The model under review builds one solid part; all positions refer to its coordinate system, in mm. A direction names the side the tool comes from. Give positions to 0.01 mm unless a question says otherwise; leave off trailing zeros. Order: outer loops, then holes, each group sorted by start corner. A loop starts at its lowest first (then second) coordinate and runs counter-clockwise, first axis right, second up. Notation, with made-up numbers: (-28, 41) - (-13, 41) arc R10 cw to (-13, 51) - close; hole circle Ø6 at (-21, -32). An arc over 180 degrees is marked (long way). Answer as CSV lines item,"result". Start each with the question number.
from build123d import *

# Parameters (mm, degrees)
SKETCH1_W           = 50
SKETCH1_H           = 265
SKETCH1_R           = 12.5
BOSS_EXTRUDE1_DEPTH = 10
SKETCH2_W           = 50
SKETCH2_H           = 20
BOSS_EXTRUDE2_DEPTH = 30
SKETCH3_W           = 50
SKETCH3_H           = 20
BOSS_EXTRUDE3_DEPTH = 30
FILLET1_R           = 10


with BuildPart() as part:
    # Sketch1 → Boss-Extrude1 (new body)
    with BuildSketch(Plane(origin=(0, 0, 0), x_dir=(1, 0, 0), z_dir=(0, 1, 0))):
        with Locations((-25, 132.5)):
            Rectangle(SKETCH1_W, SKETCH1_H)
        with Locations(Location((-25, 240, 0), (0, 0, 270))):
            Circle(SKETCH1_R, mode=Mode.SUBTRACT)
    extrude(amount=BOSS_EXTRUDE1_DEPTH)

    # Sketch2 → Boss-Extrude2 (add)
    with BuildSketch(Plane(origin=(0, 10, 0), x_dir=(1, 0, 0), z_dir=(0, 1, 0))):
        with Locations((-25, 10)):
            Rectangle(SKETCH2_W, SKETCH2_H)
    extrude(amount=BOSS_EXTRUDE2_DEPTH)

    # Sketch3 → Boss-Extrude3 (add)
    with BuildSketch(Plane.XZ):
        with Locations((-25, -10)):
            Rectangle(SKETCH3_W, SKETCH3_H)
    extrude(amount=BOSS_EXTRUDE3_DEPTH)

    # Fillet1
    fillet1_edges = [part.edges().sort_by_distance(p)[0] for p in [
        (-25, 10, -20),
        (-25, 0, -20),
    ]]
    fillet(fillet1_edges, radius=FILLET1_R)


solid = part.part
Item 1: Take a section at B-B on z = -240. Write out the cut boundary in (x, y), and give its area (3 significant figures).
Item 2: Take a section at C-C on y = 7. Write out the cut boundary in (x, z), and give its area (3 significant figures).
Item 3: Machinability: for faces 1 (the face through (-25, -20, -20)), 2 (the face through (-25, 10, -149)), 3 (the face through (-25, 5, -265)), which of the approach directions +Z, -Z, +X, -X, +Y, -Y give a long, thin tool a straight path to every point of the face, cutting with its end or side? Answer none if there is none.
Item 4: Clearance check with flat-ended pins moving along their axes: pin 1 (16 mm diameter, centred on x = -21, y = 29, fed in from -Z); pin 2 (5 mm diameter, centred on x = -8, z = -122.5, fed in from +Y); pin 3 (15 mm diameter, centred on x = -32, z = -96, fed in from -Y). State where each tip first meets the part, or that it passes through.
Item 5: Take a section at D-D on y = 23. Write out the cut boundary in (x, z).
Item 6: Mouldability with a two-part tool opening along X and no side actions: class faces 4 (the face through (-25, 5, 0)), 5 (the face through (-29.788, 4.93, -228.453)), 6 (the face through (-50, 5, -84)) as released by +X, released by -X, zero draft, split by the parting line, or undercut.
Item 7: Take a section at A-A on x = -28.5. Write out the cut boundary in (y, z), and give its area (3 significant figures).
Item 8: For line 1 along X through (y, z) = (5.25, -240); line 2 along Y through (x, z) = (-39, -116.5); line 3 along Z through (x, y) = (-18.5, -22), list the stretches that pass through material, from the lowest coordinate up.
Data:
1,outline,"(-50, 0) - (-37.5, 0) - (-37.5, 10) - (-50, 10) - close; (-12.5, 0) - (0, 0) - (0, 10) - (-12.5, 10) - close"
1,area,"250 mm^2"
2,outline,"(-50, -265) - (0, -265) - (0, 0) - (-50, 0) - close; hole circle Ø25 at (-25, -240)"
2,area,"12,800 mm^2"
3,face 1,"-Z, +X, -X, -Y"
3,face 2,"-Z, +X, -X, +Y"
3,face 3,"-Z, +X, -X, +Y, -Y"
4,pin 1,"stops at z = -20"
4,pin 2,"stops at y = 10"
4,pin 3,"stops at y = 0"
5,outline,"(-50, -20) - (0, -20) - (0, 0) - (-50, 0) - close"
6,face 4,"zero draft"
6,face 5,"undercut"
6,face 6,"released by -X"
7,outline,"(-30, -20) - (-10, -20) arc R10 cw to (0, -30) - (0, -228) - (10, -228) - (10, -30) arc R10 cw to (20, -20) - (40, -20) - (40, 0) - (-30, 0) - close; (0, -265) - (10, -265) - (10, -252) - (0, -252) - close"
7,area,"3,650 mm^2"
8,line 1,"x = -50 to -37.5, -12.5 to 0"
8,line 2,"y = 0 to 10"
8,line 3,"z = -20 to 0"
